Geometry: final body of the model. Coordinates: model frame, mm. Face numbers are marked on the shaded views. A direction names the side the tool comes from. Round coordinates to 2 decimals unless told otherwise and drop trailing zeros. Write each loop counter-clockwise with the first axis right and the second up, starting at its lowest first coordinate (ties: lowest second). Pieces come first, ordered by that corner, then holes. Notation, with made-up numbers: M -20.5,14.5 L 17.5,14.5 A23 ccw 17.5,38.5 Z; hole C 48.5,-9 d7. An arc over 180 degrees is marked long. Answer as CSV lines item,"result". Start each with the question number.
Q1. First-contact query: pin 1 (0.9 mm diameter, centred on x = -0.5, z = 0.5, fed in from +Y). Flat tip, straight axial feed; report the tip coordinate or a pass-through.
Q2. Reachability of the marked faces 1 and 2 from +Z, -Z, +X, -X, +Y, -Y: full face, straight path, thin tool, end or side. Return the list, or none.
Q3. Section query B-B on y = 3.25. Output: boundary loops of the cut face in (x, z).
Q4. Section query A-A on x = 14. Output: boundary loops of the cut face in (y, z), and give its area (3 significant figures).
Q5. Section query C-C on x = 1. Output: boundary loops of the cut face in (y, z).
Q6. Section query D-D on z = 0.75. Give the number of separate pieces and of enclosed holes in the cut face, and give its area (3 significant figures).
Q7. Mould query, pull axis Z, two halves, no side actions, for the marked faces 3, 4 and 5. Classes: pulls with the +Z half, pulls with the -Z half, needs draft (parallel to the pull), parting line crosses it, or undercut.
Q8. Ray query, probe 1 along X at (y, z) = (2.25, 0); probe 2 along Z at (x, y) = (-14, 3); probe 3 along Z at (x, y) = (13, 3.75). Return the intervals inside material, ascending.
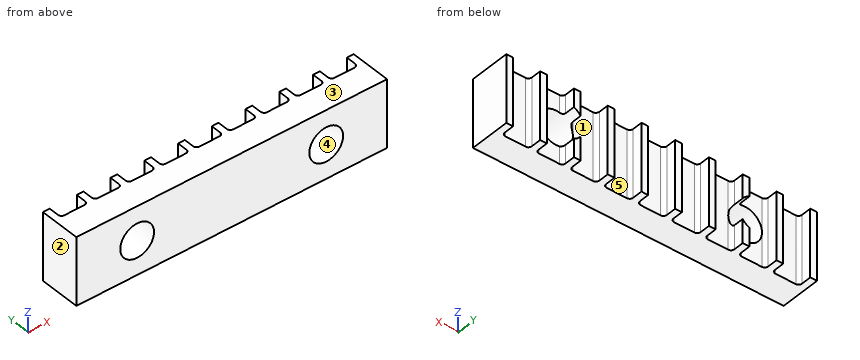
```python
from build123d import *

# Parameters (mm, degrees)
SKETCH1_W           = 46
SKETCH1_H           = 10
SKETCH1_R           = 2.5
BOSS_EXTRUDE1_DEPTH = 6
SKETCH2_W           = 4
SKETCH2_H           = 2
CUT_EXTRUDE1_DEPTH  = 26.787593916
FILLET2_R           = 0.5


with BuildPart() as part:
    # Sketch1 → Boss-Extrude1 (new body)
    with BuildSketch(Plane(origin=(0, 0, 0), x_dir=(1, 0, 0), z_dir=(0, 1, 0))):
        Rectangle(SKETCH1_W, SKETCH1_H)
        with Locations(Location((14, 0, 0), (0, 0, 270))):
            Circle(SKETCH1_R, mode=Mode.SUBTRACT)
        with Locations(Location((-14, 0, 0), (0, 0, 270))):
            Circle(SKETCH1_R, mode=Mode.SUBTRACT)
    extrude(amount=BOSS_EXTRUDE1_DEPTH)

    # Sketch2 → Cut-Extrude1 (cut, through all)
    with BuildSketch(Plane.XY.offset(5)):
        with Locations((-20, 5)):
            Rectangle(SKETCH2_W, SKETCH2_H)
        with Locations((-15, 5)):
            Rectangle(SKETCH2_W, SKETCH2_H)
        with Locations((-10, 5)):
            Rectangle(SKETCH2_W, SKETCH2_H)
        with Locations((-5, 5)):
            Rectangle(SKETCH2_W, SKETCH2_H)
        with Locations((0, 5)):
            Rectangle(SKETCH2_W, SKETCH2_H)
        with Locations((5, 5)):
            Rectangle(SKETCH2_W, SKETCH2_H)
        with Locations((10, 5)):
            Rectangle(SKETCH2_W, SKETCH2_H)
        with Locations((15, 5)):
            Rectangle(SKETCH2_W, SKETCH2_H)
        with Locations((20, 5)):
            Rectangle(SKETCH2_W, SKETCH2_H)
    extrude(amount=-CUT_EXTRUDE1_DEPTH, mode=Mode.SUBTRACT)

    # Fillet2
    fillet2_edges = [part.edges().sort_by_distance(p)[0] for p in [
        (3, 4, 0),
        (7, 4, 0),
        (8, 4, 0),
        (12, 4, 3.25),
        (12, 4, -3.25),
        (13, 4, -3.645643924),
        (13, 4, 3.645643924),
        (17, 4, 0),
        (18, 4, 0),
        (22, 4, 0),
        (-18, 4, 0),
        (-22, 4, 0),
        (-13, 4, 3.645643924),
        (-13, 4, -3.645643924),
        (-17, 4, 0),
        (-12, 4, -3.25),
        (-12, 4, 3.25),
        (-8, 4, 0),
        (-7, 4, 0),
        (-3, 4, 0),
        (-2, 4, 0),
        (2, 4, 0),
    ]]
    fillet(fillet2_edges, radius=FILLET2_R - 0.0001)  # a hair under: the kernel refuses the full size


solid = part.part
```
Entries:
1,pin 1,"stops at y = 4"
2,face 1,"+Z, -Z, +Y"
2,face 2,"+Z, -Z, -X, +Y, -Y"
3,outline,"M -23,-5 L 23,-5 L 23,5 L -23,5 Z; hole C -14,0 d5; hole C 14,0 d5"
4,outline,"M 0,-5 L 4,-5 L 4,-2.5 L 0,-2.5 Z; M 0,2.5 L 4,2.5 L 4,5 L 0,5 Z"
4,area,"20.0 mm^2"
5,outline,"M 0,-5 L 4,-5 L 4,5 L 0,5 Z"
6,separate pieces,"3"
6,enclosed holes,"0"
6,area,"163 mm^2"
7,face 3,"pulls with the +Z half"
7,face 4,"undercut"
7,face 5,"needs draft"
8,probe 1,"x = -23 to -16.5, -11.5 to 11.5, 16.5 to 23"
8,probe 2,"z = -5 to -2.5, 2.5 to 5"
8,probe 3,"z = -5 to -2.29, 2.29 to 5"
